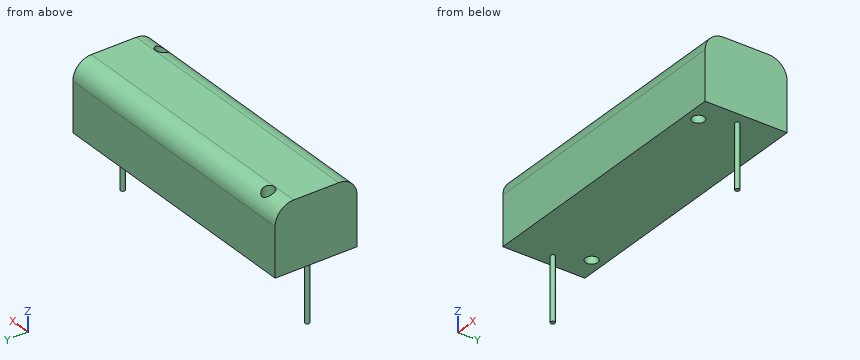
Solid Edge part; units mm, degrees
sketch "Sketch1" plane through (0, 0, 0) normal (1, 0, 0) x (0, 1, 0)
  arc A0 (-4.6355, 13.8938) -> (-8.4455, 10.0838) centre (-4.6355, 10.0838) ccw
  line L0 (-8.4455, 10.0838) -> (-8.4455, 0)
  line L1 (-8.4455, 0) -> (8.4455, 0)
  line L2 (8.4455, 0) -> (8.4455, 10.0838)
  arc A1 (4.6355, 13.8938) -> (8.4455, 10.0838) centre (4.6355, 10.0838) cw
  line L3 (4.6355, 13.8938) -> (-4.6355, 13.8938)
extrude "Protrusion1" add sketch "Sketch1" along normal blind 56.9976
sketch "Sketch2" plane through (28.4988, 0, 0) normal (0, 0, -1) x (0, 1, 0)
  circle A0 centre (0, 25.9969) radius 0.4445
  circle A1 centre (0, -25.9969) radius 0.4445
extrude "ExtrudedProtrusion_2" add sketch "Sketch2" along normal blind 13.0048
sketch "Sketch3" plane through (28.4988, 0, 0) normal (0, 0, -1) x (1, 0, 0)
  circle A0 centre (-23.241, -5.9944) radius 1.27
  circle A1 centre (23.241, 5.9944) radius 1.27
extrude "Cutout1" cut sketch "Sketch3" against normal through all
Build history of the part. All positions in model axes, mm. Round coordinates to 2 decimals unless told otherwise and drop trailing zeros. Write each loop counter-clockwise with the first axis right and the second up, starting at its lowest first coordinate (ties: lowest second). Pieces come first, ordered by that corner, then holes.
1) Band-saw the part on B-B, the plane z = -7.75. List the corners of the cut face in (x, y).
2) Band-saw the part on C-C, the plane y = 4. List the corners of the cut face in (x, z).
3) Pin check, flat tips, straight feed: pin 1 (5 mm diameter, centred on x = 22, y = -3.5, fed in from -Z); pin 2 (2 mm diameter, centred on y = 3.5, z = 0, fed in from -X); pin 3 (1.5 mm diameter, centred on x = 51.74, y = -5.99, fed in from +Z). Stop position of each tip, or through.
4) Drill centre lines: probe 1 along X at (y, z) = (-7, 6.25); probe 2 along Z at (x, y) = (17.5, 1); probe 3 along X at (y, z) = (-5.5, 7.25). Where is each one in solid material? Low to high.
5) Band-saw the part on A-A, the plane x = 5.5. List the corners of the cut face in (y, z).
Ans:
1. outline: circle Ø0.89 at (2.5, 0); circle Ø0.89 at (54.5, 0)
2. outline: (0, 0) - (57, 0) - (57, 13.89) - (0, 13.89) - close
3. pin 1: stops at z = 0
3. pin 2: stops at x = 0
3. pin 3: passes through
4. probe 1: x = 0 to 50.96, 52.52 to 57
4. probe 2: z = 0 to 13.89
4. probe 3: x = 0 to 50.57, 52.91 to 57
5. outline: (-8.45, 0) - (4.75, 0) - (4.75, 13.89) arc R3.81 ccw to (4.64, 13.89) - (-4.64, 13.89) arc R3.81 ccw to (-8.45, 10.08) - close; (7.24, 0) - (8.45, 0) - (8.45, 10.08) arc R3.81 ccw to (7.24, 12.86) - close
